Geometry check sheet. Reference: the model listing, model coordinates, mm. A direction names the side the tool comes from. Round coordinates to 2 decimals unless told otherwise and drop trailing zeros. Loops run counter-clockwise (first coordinate to the right, second up) from the corner with the lowest first, then second, coordinate; pieces in that order, holes last. Notation, with made-up numbers: (-34, 35.25) - (-26, 35.25) arc R12 ccw to (-26, 40.25) - close; hole circle Ø11 at (-35, 44). An arc over 180 degrees is marked (long way). Write item = value, one per line.
```python
from build123d import *

# Parameters (mm, degrees)
SKETCH1_R           = 3.175
BOSS_EXTRUDE1_DEPTH = 14.478
SKETCH2_R           = 38.1
BOSS_EXTRUDE2_DEPTH = 143.891
SKETCH3_W           = 2.54
SKETCH3_H           = 5.08
BOSS_EXTRUDE3_DEPTH = 14.478
SKETCH4_R           = 5.999533244
BOSS_EXTRUDE4_DEPTH = 5.08
SKETCH5_R           = 6.35
BOSS_EXTRUDE5_DEPTH = 31.75
SKETCH6_R           = 12.7
BOSS_EXTRUDE6_DEPTH = 12.7


with BuildPart() as part:
    # Sketch1 → Boss-Extrude1 (new body)
    with BuildSketch(Plane.XY):
        Circle(SKETCH1_R)
    extrude(amount=BOSS_EXTRUDE1_DEPTH)

    # Sketch2 → Boss-Extrude2 (add)
    with BuildSketch(Plane.XY.offset(14.478)):
        Circle(SKETCH2_R)
    extrude(amount=BOSS_EXTRUDE2_DEPTH)

    # Sketch3 → Boss-Extrude3 (add)
    with BuildSketch(Plane(origin=(0, 0, 0), x_dir=(-1, 0, 0), z_dir=(0, 0, -1))):
        with Locations((0, 3.175)):
            Rectangle(SKETCH3_W, SKETCH3_H)
    extrude(amount=-BOSS_EXTRUDE3_DEPTH)

    # Sketch4 → Boss-Extrude4 (add)
    with BuildSketch(Plane(origin=(0, 0, 0), x_dir=(-1, 0, 0), z_dir=(0, 0, -1))):
        Circle(SKETCH4_R)
    extrude(amount=BOSS_EXTRUDE4_DEPTH)

    # Sketch5 → Boss-Extrude5 (add)
    with BuildSketch(Plane.XY.offset(158.369)):
        Circle(SKETCH5_R)
    extrude(amount=BOSS_EXTRUDE5_DEPTH)

    # Sketch6 → Boss-Extrude6 (add)
    with BuildSketch(Plane.XY.offset(190.119)):
        Circle(SKETCH6_R)
    extrude(amount=BOSS_EXTRUDE6_DEPTH)


solid = part.part
```
(1) Gauge pin test, flat ends, axial feed: pin 1 (2 mm diameter, centred on y = 20, z = 60.5, fed in from -X); pin 2 (10 mm diameter, centred on x = 10.5, z = 58.5, fed in from -Y); pin 3 (8 mm diameter, centred on x = 7, z = 100, fed in from +Y). Record the tip position at first contact, or that the pin passes through.
Answers follow:
pin_1 = -33.02
pin_2 = -37.7
pin_3 = 37.98
(2) Scan lines: L1, parallel to Z at x = -4.5, y = 11; L2, parallel to Z at x = -30.5, y = 20; L3, parallel to Y at x = 20.5, z = 59. Record each from-to range of solid material in increasing order. Write a range as [from, to].
Answers follow:
L1 = [14.48, 158.37], [190.12, 202.82]
L2 = [14.48, 158.37]
L3 = [-32.11, 32.11]
(3) Section check C-C (x = -27). Enter the section's corners in (y, z), then the cut area to 3 significant figures.
Answers follow:
outline = (-26.88, 14.48) - (26.88, 14.48) - (26.88, 158.37) - (-26.88, 158.37) - close
area = 7,740 mm²
(4) Section check D-D (z = 173.5). Enter the section's corners in (x, y), then the cut area to 3 significant figures.
Answers follow:
outline = circle Ø12.7 at (0, 0)
area = 127 mm²
(5) Set-up check for faces 1 (the cylindrical face through (-30.235, -23.183, 85.416)), 2 (the cylindrical face through (-1.38, -6.2, 174.02)), 3 (the cylindrical face through (-2.75, -12.4, 196.38)): record each of +Z, -Z, +X, -X, +Y, -Y from which the full face is reachable in a straight line by a thin tool's end or side.
Answers follow:
face_1 = +Z, -Z
face_2 = none
face_3 = +Z
(6) Mould release check, pull along Z, two halves, no side actions. Record for faces 4 (the flat face through (3, 6, 190.119)), 5 (the cylindrical face through (1.301, -5.857, -2.504)), 6 (the flat face through (0, 0, -5.08)), 7 (the flat face through (0, 0, 202.819)): pulls with the +Z half, pulls with the -Z half, needs draft (parallel to the pull), parting line crosses it, or undercut.
Answers follow:
face_4 = undercut
face_5 = needs draft
face_6 = pulls with the -Z half
face_7 = pulls with the +Z half
(7) Section check B-B (z = 89). Enter the section's corners in (x, y), then the cut area to 3 significant figures.
Answers follow:
outline = circle Ø76.2 at (0, 0)
area = 4,560 mm²
(8) Section check A-A (y = 0). Enter the section's corners in (x, z) (3 decimals), then the cut area to 3 significant figures.
Answers follow:
outline = (-38.1, 14.478) - (-3.175, 14.478) - (-3.175, 0) - (-6, 0) - (-6, -5.08) - (6, -5.08) - (6, 0) - (3.175, 0) - (3.175, 14.478) - (38.1, 14.478) - (38.1, 158.369) - (6.35, 158.369) - (6.35, 190.119) - (12.7, 190.119) - (12.7, 202.819) - (-12.7, 202.819) - (-12.7, 190.119) - (-6.35, 190.119) - (-6.35, 158.369) - (-38.1, 158.369) - close
area = 11,800 mm²
